Autodesk Inventor part; units mm, degrees
ref_plane "YZ Plane" through (0, 0, 0) normal (1, 0, 0) x (0, 1, 0)
ref_plane "XZ Plane" through (0, 0, 0) normal (0, 1, 0) x (-1, 0, 0)
ref_plane "XY Plane" through (0, 0, 0) normal (0, 0, 1) x (1, 0, 0)
sketch "Esboço1" plane through (0, 0, 0) normal (0, 1, 0) x (-1, 0, 0)
  line L0 (127.6443, 137.7783) -> (-125.3557, 137.7783)
  line L1 (-125.3557, 137.7783) -> (-125.3557, -188.2217)
  line L2 (-125.3557, -188.2217) -> (127.6443, -188.2217)
  line L3 (127.6443, -188.2217) -> (127.6443, 137.7783)
  point P0 (0, 0)
  dimension "d0" = 326
  dimension "d1" = 253
extrude "Extrusão1" add sketch "Esboço1" along normal blind 12
sketch "Esboço2" plane through (0, 12, 0) normal (0, 1, 0) x (1, 0, 0)
  line L0 (-115.6443, -128.7783) -> (113.3557, -128.7783)
  line L1 (113.3557, -128.7783) -> (113.3557, 179.2217)
  line L2 (113.3557, 179.2217) -> (-115.6443, 179.2217)
  line L3 (-115.6443, 179.2217) -> (-115.6443, -128.7783)
  line L4 (-127.6443, -137.7783) -> (125.3557, -137.7783)
  line L5 (125.3557, 188.2217) -> (-127.6443, 188.2217)
  line L6 (-127.6443, 188.2217) -> (-127.6443, -137.7783)
  line L7 (125.3557, -137.7783) -> (125.3557, 188.2217)
  point P0 (0, 0)
  dimension "d4" = 9
  dimension "d5" = 9
  dimension "d6" = 12
  dimension "d7" = 12
extrude "Extrusão2" cut sketch "Esboço2" against normal blind 2 contours L3 L2 L1 L0
properties part number "tela"
Source: CAD feature listing. Evaluate the final solid. Frame: model axes, mm. Round coordinates to 2 decimals unless told otherwise and drop trailing zeros. Loops run counter-clockwise (first coordinate to the right, second up) from the corner with the lowest first, then second, coordinate; pieces in that order, holes last.
1. Contact query for flat-ended pins moving along their axis: pin 1 (12 mm diameter, centred on x = -11, z = -97.5, fed in from +Y); pin 2 (12 mm diameter, centred on x = -58.5, z = -137, fed in from -Y). Output: stop coordinate, or through.
2. Ray query, L1, parallel to X at y = 11, z = 39; L2, parallel to Y at x = 102, z = 72.5. Return the intervals inside material, ascending.
3. Section query B-B on x = 32.5. Output: boundary loops of the cut face in (y, z).
4. Mould query, pull axis X, two halves, no side actions, for faces 1 (the flat face through (125.356, 6, -23)), 2 (the flat face through (-3, 10, -27)), 3 (the flat face through (1, 6, -188.222)), 4 (the flat face through (-127.644, 6, -28)). Classes: released by +X, released by -X, zero draft, split by the parting line, or undercut.
5. Section query A-A on z = 112. Output: boundary loops of the cut face in (x, y), and give its area (3 significant figures).
Answers below:
1. pin 1: stops at y = 10
1. pin 2: stops at y = 0
2. L1: x = -127.64 to -115.64, 113.36 to 125.36
2. L2: y = 0 to 10
3. outline: (0, -188.22) - (12, -188.22) - (12, -179.22) - (10, -179.22) - (10, 128.78) - (12, 128.78) - (12, 137.78) - (0, 137.78) - close
4. face 1: released by +X
4. face 2: undercut
4. face 3: zero draft
4. face 4: released by -X
5. outline: (-127.64, 0) - (125.36, 0) - (125.36, 12) - (113.36, 12) - (113.36, 10) - (-115.64, 10) - (-115.64, 12) - (-127.64, 12) - close
5. area: 2,580 mm2
